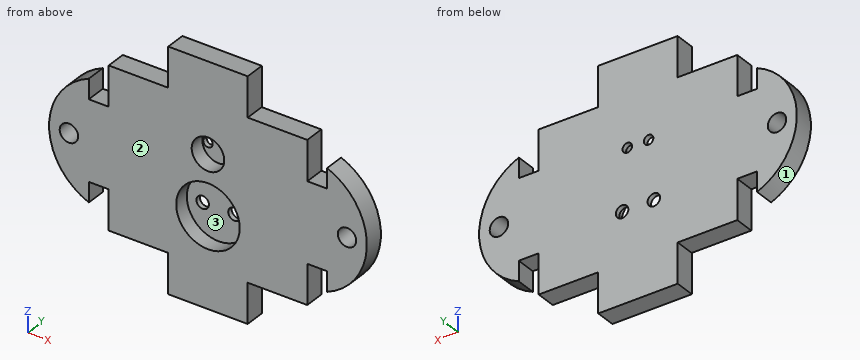
```python
from build123d import *

# Parameters (mm, degrees)
BOSS_EXTRUDE1_DEPTH       = 3.175
F_4_CLEARANCE_HOLE1_D     = 2.9464
F_4_CLEARANCE_HOLE1_DEPTH = 6.35
F_4_CLEARANCE_HOLE1_TIP   = 0.885187864
CUT_EXTRUDE3_REACH        = 5.175
SKETCH4_R                 = 0.762
SKETCH4_R_2               = 1
SKETCH4_3_R               = 2.6035
SKETCH4_3_R_2             = 0.762
SKETCH4_3_R_3             = 5.08
SKETCH4_3_R_4             = 1
CUT_EXTRUDE4_DEPTH        = 2.4


with BuildPart() as part:
    # Sketch1 → Boss-Extrude1 (new body)
    with BuildSketch(Plane(origin=(0, 0, 0), x_dir=(1, 0, 0), z_dir=(0, 1, 0))):
        with BuildLine():
            Line((-15.875, 12.7), (-6.35, 12.7))
            Line((-6.35, 12.7), (-6.35, 19.05))
            Line((-6.35, 19.05), (6.35, 19.05))
            Line((6.35, 19.05), (6.35, 12.7))
            Line((6.35, 12.7), (15.875, 12.7))
            Line((15.875, 12.7), (15.875, 6.35))
            Line((15.875, 6.35), (19.05, 6.35))
            Line((19.05, 6.35), (19.05, 9.525))
            ThreePointArc((19.05, 9.525), (25.4, 0), (19.05, -9.525))
            Line((19.05, -9.525), (19.05, -6.35))
            Line((19.05, -6.35), (15.875, -6.35))
            Line((15.875, -6.35), (15.875, -12.7))
            Line((15.875, -12.7), (6.35, -12.7))
            Line((6.35, -12.7), (6.35, -19.05))
            Line((6.35, -19.05), (-6.35, -19.05))
            Line((-6.35, -19.05), (-6.35, -12.7))
            Line((-6.35, -12.7), (-15.875, -12.7))
            Line((-15.875, -12.7), (-15.875, -6.35))
            Line((-15.875, -6.35), (-19.05, -6.35))
            Line((-19.05, -6.35), (-19.05, -9.525))
            ThreePointArc((-19.05, -9.525), (-25.4, 0), (-19.05, 9.525))
            Line((-19.05, 9.525), (-19.05, 6.35))
            Line((-19.05, 6.35), (-15.875, 6.35))
            Line((-15.875, 6.35), (-15.875, 12.7))
        make_face()
    extrude(amount=BOSS_EXTRUDE1_DEPTH)

    # 4 Clearance Hole1
    with Locations(Plane(origin=(0, 3.175, 0), x_dir=(-1, 0, 0), z_dir=(0, 1, 0))):
        with Locations((-22.225, 0), (22.225, 0)):
            Hole(F_4_CLEARANCE_HOLE1_D / 2, depth=F_4_CLEARANCE_HOLE1_DEPTH)
            with Locations((0, 0, -(F_4_CLEARANCE_HOLE1_DEPTH + F_4_CLEARANCE_HOLE1_TIP / 2))):  # 118° drill point
                Cone(0, F_4_CLEARANCE_HOLE1_D / 2, F_4_CLEARANCE_HOLE1_TIP, mode=Mode.SUBTRACT)

    # Sketch4 → Cut-Extrude3 (cut, up to next)
    with BuildSketch(Plane(origin=(0, 0, 0), x_dir=(1, 0, 0), z_dir=(0, 1, 0)), mode=Mode.PRIVATE) as cut_extrude3_sk1:
        with Locations((-1.7, -4.7625)):
            Circle(SKETCH4_R)
    cut_extrude3_tool1 = extrude(cut_extrude3_sk1.sketch, amount=CUT_EXTRUDE3_REACH, mode=Mode.PRIVATE) & part.part
    add(cut_extrude3_tool1.solids().sort_by_distance((-1.7, 0, 4.7625))[0], mode=Mode.SUBTRACT)
    # Sketch4 → Cut-Extrude3 (cut, up to next)
    with BuildSketch(Plane(origin=(0, 0, 0), x_dir=(1, 0, 0), z_dir=(0, 1, 0)), mode=Mode.PRIVATE) as cut_extrude3_sk2:
        with Locations((1.7, -4.7625)):
            Circle(SKETCH4_R)
    cut_extrude3_tool2 = extrude(cut_extrude3_sk2.sketch, amount=CUT_EXTRUDE3_REACH, mode=Mode.PRIVATE) & part.part
    add(cut_extrude3_tool2.solids().sort_by_distance((1.7, 0, 4.7625))[0], mode=Mode.SUBTRACT)
    # Sketch4 → Cut-Extrude3 (cut, up to next)
    with BuildSketch(Plane(origin=(0, 0, 0), x_dir=(1, 0, 0), z_dir=(0, 1, 0)), mode=Mode.PRIVATE) as cut_extrude3_sk3:
        with Locations((2.54, 4.7625)):
            Circle(SKETCH4_R_2)
    cut_extrude3_tool3 = extrude(cut_extrude3_sk3.sketch, amount=CUT_EXTRUDE3_REACH, mode=Mode.PRIVATE) & part.part
    add(cut_extrude3_tool3.solids().sort_by_distance((2.54, 0, -4.7625))[0], mode=Mode.SUBTRACT)
    # Sketch4 → Cut-Extrude3 (cut, up to next)
    with BuildSketch(Plane(origin=(0, 0, 0), x_dir=(1, 0, 0), z_dir=(0, 1, 0)), mode=Mode.PRIVATE) as cut_extrude3_sk4:
        with Locations((-2.54, 4.7625)):
            Circle(SKETCH4_R_2)
    cut_extrude3_tool4 = extrude(cut_extrude3_sk4.sketch, amount=CUT_EXTRUDE3_REACH, mode=Mode.PRIVATE) & part.part
    add(cut_extrude3_tool4.solids().sort_by_distance((-2.54, 0, -4.7625))[0], mode=Mode.SUBTRACT)

    # Sketch4_3 → Cut-Extrude4 (cut)
    with BuildSketch(Plane(origin=(0, 0, 0), x_dir=(1, 0, 0), z_dir=(0, 1, 0))):
        with Locations((0, -4.7625)):
            Circle(SKETCH4_3_R)
        with Locations((-1.7, -4.7625)):
            Circle(SKETCH4_3_R_2, mode=Mode.SUBTRACT)
        with Locations((1.7, -4.7625)):
            Circle(SKETCH4_3_R_2, mode=Mode.SUBTRACT)
        with Locations((1.7, -4.7625)):
            Circle(SKETCH4_3_R_2)
        with Locations((0, 4.7625)):
            Circle(SKETCH4_3_R_3)
        with Locations((2.54, 4.7625)):
            Circle(SKETCH4_3_R_4, mode=Mode.SUBTRACT)
        with Locations((-2.54, 4.7625)):
            Circle(SKETCH4_3_R_4, mode=Mode.SUBTRACT)
    extrude(amount=CUT_EXTRUDE4_DEPTH, mode=Mode.SUBTRACT)


solid = part.part
```
Can you work these out from the model? Positions are in its coordinate system, mm. Face numbers are marked on the shaded views. Round coordinates to 2 decimals unless told otherwise and drop trailing zeros. Loops run counter-clockwise (first coordinate to the right, second up) from the corner with the lowest first, then second, coordinate; pieces in that order, holes last.
Item 1: Suppose I cut it at D-D, the plane z = 14. Write out the boundary of the cut face in (x, y) (3 decimals), then the cut area to 3 significant figures.
Item 2: Suppose I cut it at C-C, the plane z = -8. Write out the boundary of the cut face in (x, y) (3 decimals).
Item 3: Will these pins go through, and if not, where does the flat tip stop? pin 1 Ø1 at (y, z) = (2, -8) entering from -X; pin 2 Ø2.5 at (x, z) = (0.5, 5) entering from -Y; pin 3 Ø2.5 at (x, z) = (-22.225, 0) entering from +Y; pin 4 Ø1.6 at (y, z) = (1.5, -8) entering from +X.
Item 4: Please list where these lines run through material, in increasing order: L1, parallel to Z at x = 0, y = 1.65; L2, parallel to X at y = 1.8, z = -8 (3 decimals); L3, parallel to Z at x = -2.54, y = 2.6.
Item 5: If we mould it in two halves opening along X, with no side actions, what happens to the marked faces 1, 2 and 3? For each: +X half, -X half, draft (parallel to the pull), parting line (faces both ways), or undercut.
Item 6: Suppose I cut it at A-A, the plane y = 1.9. State how many separate pieces and enclosed holes the cut face has, then the cut area to 3 significant figures.
Reported:
1. outline: (-6.35, 0) - (6.35, 0) - (6.35, 3.175) - (-6.35, 3.175) - close
1. area: 40.3 mm2
2. outline: (-21.599, 0) - (-19.05, 0) - (-19.05, 3.175) - (-21.599, 3.175) - close; (-15.875, 0) - (-3.915, 0) - (-3.915, 2.4) - (3.915, 2.4) - (3.915, 0) - (15.875, 0) - (15.875, 3.175) - (-15.875, 3.175) - close; (19.05, 0) - (21.599, 0) - (21.599, 3.175) - (19.05, 3.175) - close
3. pin 1: stops at x = -22.17
3. pin 2: stops at y = 2.4
3. pin 3: passes through
3. pin 4: stops at x = 22.47
4. L1: z = -19.05 to -9.84, 0.32 to 2.16, 7.37 to 19.05
4. L2: x = -21.599 to -19.05, -15.875 to -3.915, 3.915 to 15.875, 19.05 to 21.599
4. L3: z = -19.05 to -5.76, -3.76 to 19.05
5. face 1: -X half
5. face 2: draft
5. face 3: undercut
6. separate pieces: 1
6. enclosed holes: 4
6. area: 1,110 mm2
